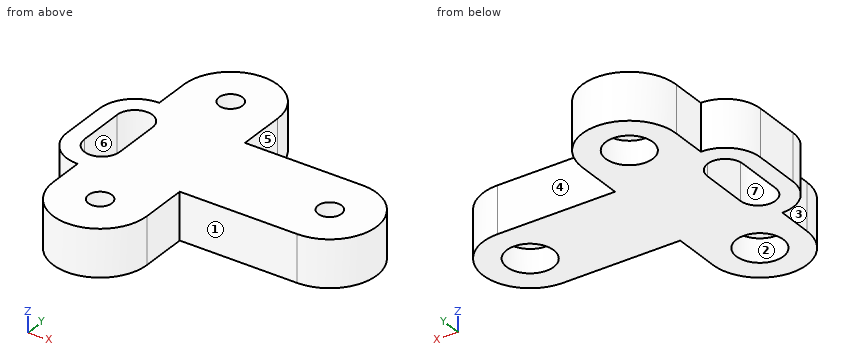
Autodesk Fusion 360 part; units mm, degrees
sketch "Sketch1" plane through (0, 0, 0) normal (0, 0, 1) x (1, 0, 0)
  circle A0 centre (0, 80) radius 10
  circle A1 centre (0, 80) radius 15
  circle A2 centre (70, 40) radius 10
  circle A3 centre (70, 40) radius 15
  circle A4 centre (0, 0) radius 10
  circle A5 centre (0, 0) radius 15
  line L0 (20, 60) -> (70, 60)
  arc A6 (20, 80) -> (-20, 80) centre (0, 80) ccw
  arc A7 (-20, 0) -> (20, 0) centre (0, 0) ccw
  line L1 (20, 20) -> (70, 20)
  arc A8 (70, 20) -> (70, 60) centre (70, 40) ccw
  line L2 (20, 80) -> (20, 60)
  line L3 (20, 20) -> (20, 0)
  line L4 (-35, 50) -> (-35, 30)
  arc A9 (-35, 30) -> (-20, 15) centre (-20, 30) ccw
  arc A10 (-20, 65) -> (-35, 50) centre (-20, 50) ccw
  line L5 (-20, 80) -> (-20, 65)
  line L6 (-20, 15) -> (-20, 0)
  line L7 (-12.5, 50) -> (-12.5, 30)
  line L8 (-27.5, 50) -> (-27.5, 30)
  arc A11 (-12.5, 50) -> (-27.5, 50) centre (-20, 50) ccw
  arc A12 (-27.5, 30) -> (-12.5, 30) centre (-20, 30) ccw
  dimension "d1" = 20
  dimension "d2" = 30
  dimension "d3" = 40
  dimension "d4" = 20
  dimension "d5" = 30
  dimension "d6" = 40
  dimension "d7" = 20
  dimension "d8" = 30
  dimension "d9" = 40
  dimension "d10" = 80
  dimension "d11" = 40
  dimension "d12" = 70
  dimension "d13" = 40
  dimension "d14" = 20
  dimension "d16" = 30
  dimension "d18" = 30
  dimension "d19" = 20
  dimension "d20" = 20
  dimension "d21" = 30
  dimension "d22" = 15
  dimension "d23" = 15
  dimension "d24" = 20
  dimension "d25" = 30
  dimension "d27" = 12.5
  dimension "d28" = 27.5
extrude "Extrude1" add sketch "Sketch1" along normal mid plane 20 contours A1 | A3 | A5 | L0 A6 A7 L1 A8 L2 L3 L4 A9 A10 L5 L6
sketch "Sketch2" plane through (0, 0, 10) normal (0, 0, 1) x (1, 0, 0)
  circle A0 centre (0, 0) radius 10
  circle A1 centre (0, 80) radius 10
  circle A2 centre (70, 40) radius 10
  arc A3 (-12.5, 50) -> (-27.5, 50) centre (-20, 50) ccw
  line L0 (-12.5, 50) -> (-12.5, 30)
  arc A4 (-27.5, 30) -> (-12.5, 30) centre (-20, 30) ccw
  line L1 (-27.5, 30) -> (-27.5, 50)
  arc A5 (20, 80) -> (-20, 80) centre (0, 80) ccw
  line L2 (-20, 80) -> (-20, 65)
  arc A6 (-20, 65) -> (-35, 50) centre (-20, 50) ccw
  line L3 (-35, 50) -> (-35, 30)
  arc A7 (-35, 30) -> (-20, 15) centre (-20, 30) ccw
  line L4 (-20, 15) -> (-20, 0)
  arc A8 (-20, 0) -> (20, 0) centre (0, 0) ccw
  line L5 (20, 0) -> (20, 20)
  line L6 (20, 20) -> (70, 20)
  arc A9 (70, 20) -> (70, 60) centre (70, 40) ccw
  line L7 (70, 60) -> (20, 60)
  line L8 (20, 60) -> (20, 80)
  circle A10 centre (0, 80) radius 5
  circle A11 centre (70, 40) radius 5
  circle A12 centre (0, 0) radius 5
  dimension "d31" = 10
  dimension "d32" = 10
  dimension "d33" = 10
extrude "Extrude2" add sketch "Sketch2" against normal blind 10 contours A0 | A1 | A2
Model file for the job. Use its own axes, mm. Face numbers are marked on the shaded views. A direction names the side the tool comes from. Give positions to 0.01 mm unless a question says otherwise; leave off trailing zeros. Write each loop counter-clockwise with the first axis right and the second up, starting at its lowest first coordinate (ties: lowest second). Pieces come first, ordered by that corner, then holes. Notation, with made-up numbers: (-26.75, 67) - (1.25, 67) arc R25 cw to (1.25, 80) - close; hole circle Ø2 at (89.25, 86). An arc over 180 degrees is marked (long way). One line per question, with ' | ' between items. Start each with the question number.
(1) 3-axis set-ups, long thin cutter, end or side, ignore diameter. For the marked faces 1, 2 and 3: which of +Z, -Z, +X, -X, +Y, -Y reach the whole face in a straight line?
(2) Two-plate mould, pull along Y, no slides. Class the marked faces 4, 5, 6 and 7: +Y half, -Y half, draft (parallel to the pull), parting line (faces both ways), or undercut.
(3) Slice it at B-B on x = 0. Write the cut outline in (y, z).
(4) Slice it at D-D on x = 67. Write the cut outline in (y, z), plus the area to 3 significant figures.
(5) Wall check: line 1 along Y through (x, z) = (0, -2.5); line 2 along Y through (x, z) = (0, 4.75); line 3 along Y through (x, z) = (64, 3.75). Give the ranges that are in metal, low to high. Write a range as from..to.
(6) Slice it at A-A on y = 40. Write the cut outline in (x, z), plus the area to 3 significant figures.
(7) Pin check, flat tips, straight feed: P1, Ø2, axis at x = -12.5, z = 7.5, coming from the -Y side; P2, Ø4.5, axis at y = 76, z = 3, coming from the -X side; P3, Ø13, axis at x = 0, y = 80, coming from the -Z side. Stop position of each tip, or through.
(8) Slice it at C-C on z = -5.5. Write the cut outline in (x, y).
Results below:
1) face 1: +Z, -Z, +X, -Y | face 2: -Z | face 3: +Z, -Z, -X, -Y
2) face 4: +Y half | face 5: draft | face 6: undercut | face 7: undercut
3) outline: (-20, -10) - (-10, -10) - (-10, 0) - (-5, 0) - (-5, 10) - (-20, 10) - close; (5, 0) - (10, 0) - (10, -10) - (70, -10) - (70, 0) - (75, 0) - (75, 10) - (5, 10) - close; (85, 0) - (90, 0) - (90, -10) - (100, -10) - (100, 10) - (85, 10) - close
4) outline: (20, -10) - (30.46, -10) - (30.46, 0) - (36, 0) - (36, 10) - (20, 10) - close; (44, 0) - (49.54, 0) - (49.54, -10) - (60, -10) - (60, 10) - (44, 10) - close | area: 529 mm^2
5) line 1: -20..-10, 10..70, 90..100 | line 2: -20..-5, 5..75, 85..100 | line 3: 20..60
6) outline: (-35, -10) - (-27.5, -10) - (-27.5, 10) - (-35, 10) - close; (-12.5, -10) - (60, -10) - (60, 0) - (65, 0) - (65, 10) - (-12.5, 10) - close; (75, 0) - (80, 0) - (80, -10) - (90, -10) - (90, 10) - (75, 10) - close | area: 1,900 mm^2
7) P1: y = -16.36 | P2: x = -20 | P3: z = 0
8) outline: (-35, 30) arc R15 ccw to (-20, 15) - (-20, 0) arc R20 ccw to (20, 0) - (20, 20) - (70, 20) arc R20 ccw to (70, 60) - (20, 60) - (20, 80) arc R20 ccw to (-20, 80) - (-20, 65) arc R15 ccw to (-35, 50) - close; hole (-27.5, 30) arc R7.5 ccw to (-12.5, 30) - (-12.5, 50) arc R7.5 ccw to (-27.5, 50) - close; hole circle Ø20 at (0, 0); hole circle Ø20 at (0, 80); hole circle Ø20 at (70, 40)
